```python
from build123d import *

# Parameters (mm, degrees)
F0_W     = 85
F0_H     = 23
F0_H_2   = 40
F1_DEPTH = 3
F2_W     = 3
F2_H     = 23
F3_DEPTH = 24
F4_W     = 3
F4_H     = 23
F5_DEPTH = 25


with BuildPart() as f1:
    # F0 (on Top) → F1 (new body)
    with BuildSketch(Plane.XY):
        with Locations((42.5, 11.5)):
            Rectangle(F0_W, F0_H)
        with Locations((42.5, -20)):
            Rectangle(F0_W, F0_H_2)
    extrude(amount=F1_DEPTH)

    # F2 (on face) → F3 (join)
    with BuildSketch(Plane.XY.offset(3)):
        with Locations((1.5, 11.5)):
            Rectangle(F2_W, F2_H)
        with Locations((83.5, 11.5)):
            Rectangle(F2_W, F2_H)
    extrude(amount=F3_DEPTH)

    # F4 (on face) → F5 (join)
    with BuildSketch(Plane.XY.offset(27)):
        with Locations((1.5, 11.5)):
            Rectangle(F4_W, F4_H)
    extrude(amount=F5_DEPTH)


solid = f1.part
```
Verification items for the finished model (mm, model axes). A direction names the side the tool comes from. Give positions to 0.01 mm unless a question says otherwise; leave off trailing zeros. Write each loop counter-clockwise with the first axis right and the second up, starting at its lowest first coordinate (ties: lowest second). Pieces come first, ordered by that corner, then holes. Notation, with made-up numbers: (65, 85) - (101, 85) arc R22 ccw to (101, 108) - close; hole circle Ø9 at (-18, 11). An arc over 180 degrees is marked (long way). Put each result on its own line as item: value.
Q1. Section check C-C on x = 21. Record the cut outline in (y, z).
Result:
outline: (-40, 0) - (23, 0) - (23, 3) - (-40, 3) - close
Q2. Section check D-D on z = 36. Record the cut outline in (x, y), and give its area (3 significant figures).
Result:
outline: (0, 0) - (3, 0) - (3, 23) - (0, 23) - close
area: 69.0 mm2
Q3. Scan lines: probe 1 along X at (y, z) = (6.5, 22.5); probe 2 along Z at (x, y) = (39, -2). Record each from-to range of solid material in increasing order. Write a range as from..to.
Result:
probe 1: 0..3, 82..85
probe 2: 0..3
Q4. Mould release check, pull along X, two halves, no side actions. Record for faces 1 (the face through (85, 5, 10)), 2 (the face through (1, 12, 52)), 3 (the face through (82, 11, 15)): released by +X, released by -X, zero draft, split by the parting line, or undercut.
Result:
face 1: released by +X
face 2: zero draft
face 3: undercut
Q5. Section check A-A on z = 19.5. Record the cut outline in (x, y), and give its area (3 significant figures).
Result:
outline: (0, 0) - (3, 0) - (3, 23) - (0, 23) - close; (82, 0) - (85, 0) - (85, 23) - (82, 23) - close
area: 138 mm2
Q6. Section check B-B on y = 13. Record the cut outline in (x, z).
Result:
outline: (0, 0) - (85, 0) - (85, 27) - (82, 27) - (82, 3) - (3, 3) - (3, 52) - (0, 52) - close
Q7. Set-up check for faces 4 (the face through (3, 11, 27)), 5 (the face through (83, 0, 15)), 6 (the face through (83, 12, 27)): record each of +Z, -Z, +X, -X, +Y, -Y from which the full face is reachable in a straight line by a thin tool's end or side.
Result:
face 4: +Z, +Y, -Y
face 5: +Z, +X, -X, -Y
face 6: +Z, +X, +Y, -Y
Q8. Depth check by flat-ended pin: P1, Ø2.5, axis at x = 84, y = 8, coming from the +Z side; P2, Ø19, axis at x = 44, y = 6.5, coming from the +Z side; P3, Ø3.5, axis at x = 1.5, z = 15.5, coming from the -Y side; P4, Ø1, axis at x = 39, y = -19.5, coming from the -Z side. Enter the tip coordinate at first touch or a pass-through.
Result:
P1: z = 27
P2: z = 3
P3: y = 0
P4: z = 0
